Input: part model. Units: mm. Frame: model coordinates. A direction names the side the tool comes from. Round coordinates to 2 decimals unless told otherwise and drop trailing zeros. Loops run counter-clockwise (first coordinate to the right, second up) from the corner with the lowest first, then second, coordinate; pieces in that order, holes last. Notation, with made-up numbers: M 20,17.5 L 46,17.5 A14 ccw 46,35.5 Z; hole C 63,51 d11. An arc over 180 degrees is marked long. Put each result on its own line as item: value. Start each with the question number.
1) Pin query (flat end, axial travel): pin 1 (3.5 mm diameter, centred on x = -34, z = 30, fed in from -Y); pin 2 (8 mm diameter, centred on x = 4.5, z = 12, fed in from +Y); pin 3 (4 mm diameter, centred on x = 34, y = 9, fed in from +Z). Return the tip coordinate at first contact, or that it passes through.
2) Section B-B on y = -7.25. State how many separate pieces and enclosed holes the cut face has, plus the area to 3 significant figures.
3) Section A-A on y = 4.5. Output: boundary loops of the cut face in (x, z).
4) Reachability of faces 4 (the face through (1, -8, -12.6)), 5 (the face through (54.93, -0.51, 17.5)), 6 (the face through (1, 1.4, -23)) from +Z, -Z, +X, -X, +Y, -Y: full face, straight path, thin tool, end or side. Return the list, or none.
5) Section D-D on z = 3.5. Output: boundary loops of the cut face in (x, y), plus the area to 3 significant figures.
6) Line query: probe 1 along Z at (x, y) = (-31.5, 8.5); probe 2 along Y at (x, z) = (-29, 5.5); probe 3 along Y at (x, z) = (-65, 32). Output: solid intervals per line, ascending.
7) Draft query along Z for faces 1 (the face through (1, -8, -6.1)), 2 (the face through (-70, 0, -3)), 3 (the face through (1, -1.4, 10)). Return one class per face: +Z half, -Z half, draft (parallel to the pull), parting line (faces both ways), or undercut.
from build123d import *

# Parameters (mm, degrees)
BOSS_EXTRUDE1_DEPTH     = 70
CUT_EXTRUDE1_DEPTH      = 80.602528226
CUT_EXTRUDE1_DEPTH_BACK = 80.602528226
SKETCH2_R               = 1.5
CUT_EXTRUDE2_DEPTH      = 99.790801697
CUT_EXTRUDE2_DEPTH_BACK = 3
SKETCH3_R               = 1.5
CHAMFER1_SIZE           = 1


with BuildPart() as part:
    # Sketch1 → Boss-Extrude1 (new, symmetric)
    with BuildSketch(Plane(origin=(0, 0, 0), x_dir=(0, 0, -1), z_dir=(1, 0, 0))):
        with BuildLine():
            Line((34, 14.4), (34, -14.4))
            ThreePointArc((34, -14.4), (33.05, -15.35), (32.1, -14.4))
            Line((32.1, -14.4), (32.1, -1.4))
            Line((32.1, -1.4), (27.5, -1.4))
            Line((27.5, -1.4), (27.5, -14.4))
            ThreePointArc((27.5, -14.4), (26.55, -15.35), (25.6, -14.4))
            Line((25.6, -14.4), (25.6, -1.4))
            Line((25.6, -1.4), (21, -1.4))
            Line((21, -1.4), (21, -14.4))
            ThreePointArc((21, -14.4), (20.05, -15.35), (19.1, -14.4))
            Line((19.1, -14.4), (19.1, -1.4))
            Line((19.1, -1.4), (14.5, -1.4))
            Line((14.5, -1.4), (14.5, -14.4))
            ThreePointArc((14.5, -14.4), (13.55, -15.35), (12.6, -14.4))
            Line((12.6, -14.4), (12.6, -1.4))
            Line((12.6, -1.4), (8, -1.4))
            Line((8, -1.4), (8, -14.4))
            ThreePointArc((8, -14.4), (7.05, -15.35), (6.1, -14.4))
            Line((6.1, -14.4), (6.1, -1.4))
            Line((6.1, -1.4), (1.5, -1.4))
            Line((1.5, -1.4), (1.5, -14.4))
            ThreePointArc((1.5, -14.4), (0.55, -15.35), (-0.4, -14.4))
            Line((-0.4, -14.4), (-0.4, -1.4))
            Line((-0.4, -1.4), (-6.1, -1.4))
            Line((-6.1, -1.4), (-6.1, -14.492205882))
            ThreePointArc((-6.1, -14.492205882), (-7.05, -15.35), (-8, -14.492205882))
            Line((-8, -14.492205882), (-8, -1.4))
            Line((-8, -1.4), (-12.6, -1.4))
            Line((-12.6, -1.4), (-12.6, -14.492205882))
            ThreePointArc((-12.6, -14.492205882), (-13.55, -15.35), (-14.5, -14.492205882))
            Line((-14.5, -14.492205882), (-14.5, -1.4))
            Line((-14.5, -1.4), (-19.1, -1.4))
            Line((-19.1, -1.4), (-19.1, -14.492205882))
            ThreePointArc((-19.1, -14.492205882), (-20.05, -15.35), (-21, -14.492205882))
            Line((-21, -14.492205882), (-21, -1.4))
            Line((-21, -1.4), (-25.6, -1.4))
            Line((-25.6, -1.4), (-25.6, -14.492205882))
            ThreePointArc((-25.6, -14.492205882), (-26.55, -15.35), (-27.5, -14.492205882))
            Line((-27.5, -14.492205882), (-27.5, -5.6))
            Line((-27.5, -5.6), (-32.1, -5.6))
            Line((-32.1, -5.6), (-32.1, -14.492205882))
            ThreePointArc((-32.1, -14.492205882), (-33.05, -15.35), (-34, -14.492205882))
            Line((-34, -14.492205882), (-34, 1.4))
            Line((-34, 1.4), (-0.4, 1.4))
            Line((-0.4, 1.4), (-0.4, 14.4))
            ThreePointArc((-0.4, 14.4), (0.55, 15.35), (1.5, 14.4))
            Line((1.5, 14.4), (1.5, 1.4))
            Line((1.5, 1.4), (6.1, 1.4))
            Line((6.1, 1.4), (6.1, 14.4))
            ThreePointArc((6.1, 14.4), (7.05, 15.35), (8, 14.4))
            Line((8, 14.4), (8, 1.4))
            Line((8, 1.4), (12.6, 1.4))
            Line((12.6, 1.4), (12.6, 14.4))
            ThreePointArc((12.6, 14.4), (13.55, 15.35), (14.5, 14.4))
            Line((14.5, 14.4), (14.5, 1.4))
            Line((14.5, 1.4), (19.1, 1.4))
            Line((19.1, 1.4), (19.1, 14.4))
            ThreePointArc((19.1, 14.4), (20.05, 15.35), (21, 14.4))
            Line((21, 14.4), (21, 1.4))
            Line((21, 1.4), (25.6, 1.4))
            Line((25.6, 1.4), (25.6, 14.4))
            ThreePointArc((25.6, 14.4), (26.55, 15.35), (27.5, 14.4))
            Line((27.5, 14.4), (27.5, 1.4))
            Line((27.5, 1.4), (32.1, 1.4))
            Line((32.1, 1.4), (32.1, 14.4))
            ThreePointArc((32.1, 14.4), (33.05, 15.35), (34, 14.4))
        make_face()
    extrude(amount=BOSS_EXTRUDE1_DEPTH, both=True)

    # Sketch2 → Cut-Extrude1 (cut, two sides: drawn at the far end of the back side and taken through both)
    with BuildSketch(Plane(origin=(0, 1.4, 0), x_dir=(1, 0, 0), z_dir=(0, 1, 0)).offset(-CUT_EXTRUDE1_DEPTH_BACK)):
        with Locations(Location((55, -16, 0), (0, 0, 90))):
            Circle(SKETCH2_R)
        with Locations(Location((33, -16, 0), (0, 0, 90))):
            Circle(SKETCH2_R)
        with Locations(Location((11, -16, 0), (0, 0, 90))):
            Circle(SKETCH2_R)
        with Locations(Location((-55, -16, 0), (0, 0, 90))):
            Circle(SKETCH2_R)
        with Locations(Location((-33, -16, 0), (0, 0, 90))):
            Circle(SKETCH2_R)
        with Locations(Location((-11, -16, 0), (0, 0, 90))):
            Circle(SKETCH2_R)
    extrude(amount=CUT_EXTRUDE1_DEPTH + CUT_EXTRUDE1_DEPTH_BACK, mode=Mode.SUBTRACT)

    # Sketch3 → Cut-Extrude2 (cut, two sides: drawn at the far end of the back side and taken through both)
    with BuildSketch(Plane.XY.offset(34).offset(-CUT_EXTRUDE2_DEPTH_BACK)):
        with Locations(Location((65, -7.25, 0), (0, 0, 180))):
            Circle(SKETCH3_R)
        with Locations(Location((0, -7.25, 0), (0, 0, 180))):
            Circle(SKETCH3_R)
        with Locations(Location((-65, -7.25, 0), (0, 0, 180))):
            Circle(SKETCH3_R)
    extrude(amount=CUT_EXTRUDE2_DEPTH + CUT_EXTRUDE2_DEPTH_BACK, mode=Mode.SUBTRACT)

    # Chamfer1
    chamfer1_edges = [part.edges().sort_by_distance(p)[0] for p in [
        (55, 1.4, 17.5),
        (-11, 1.4, 17.5),
        (-33, 1.4, 17.5),
        (-55, 1.4, 17.5),
        (11, 1.4, 17.5),
        (33, 1.4, 17.5),
        (66.5, -7.25, 34),
        (1.5, -7.25, 34),
        (-63.5, -7.25, 34),
    ]]
    chamfer(chamfer1_edges, length=CHAMFER1_SIZE)


solid = part.part
Geometry results:
1. pin 1: stops at y = -5.6
1. pin 2: stops at y = 1.4
1. pin 3: stops at z = 0.4
2. separate pieces: 14
2. enclosed holes: 0
2. area: 2,910 mm²
3. outline: M -70,-34 L 70,-34 L 70,-32.1 L -70,-32.1 Z; M -70,-27.5 L 70,-27.5 L 70,-25.6 L -70,-25.6 Z; M -70,-21 L 70,-21 L 70,-19.1 L -70,-19.1 Z; M -70,-14.5 L 70,-14.5 L 70,-12.6 L -70,-12.6 Z; M -70,-8 L 70,-8 L 70,-6.1 L -70,-6.1 Z; M -70,-1.5 L 70,-1.5 L 70,0.4 L -70,0.4 Z
4. face 4: +X, -X, -Y
4. face 5: +Y, -Y
4. face 6: +X, -X, +Y
5. outline: M -70,-1.4 L 70,-1.4 L 70,1.4 L -70,1.4 Z
5. area: 392 mm²
6. probe 1: z = -34 to -32.1, -27.5 to -25.6, -21 to -19.1, -14.5 to -12.6, -8 to -6.1, -1.5 to 0.4
6. probe 2: y = -1.4 to 1.4
6. probe 3: y = -5.6 to 1.4
7. face 1: undercut
7. face 2: draft
7. face 3: undercut
